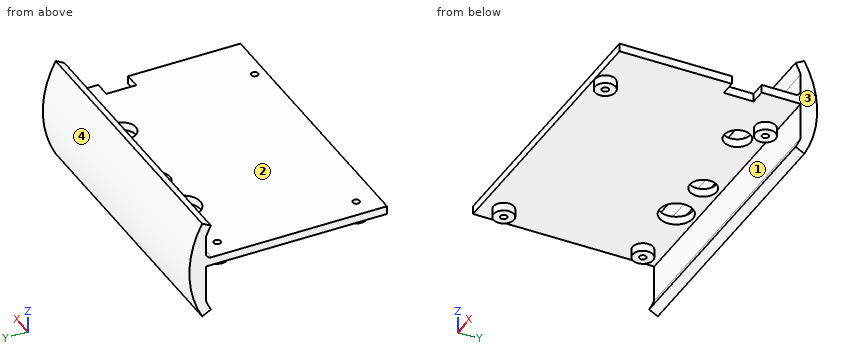
from build123d import *

# Parameters (mm, degrees)
ESBO_O1_R                                 = 5
ESBO_O1_R_2                               = 4
RESSALTO_EXTRUS_O4_DEPTH                  = 2.5
ESBO_O7_R                                 = 3.0875
RESSALTO_EXTRUS_O5_DEPTH                  = 2.5
BROCA_DE_ROSQUEAR_PARA_TARRAXA_DE_M2_51_D = 2.05
RESSALTO_EXTRUS_O6_REACH                  = 92.839


with BuildPart() as part:
    # Esboço1 → Ressalto-extrusão4 (new body)
    with BuildSketch(Plane.XY):
        Polygon((36.83, 26.550055291), (-30.48, 26.550055291), (-43.18, 26.550055291), (-43.18, 13.850055291), (-43.18, -15.359944709), (-43.18, -28.059944709), (-30.48, -28.059944709), (36.83, -28.059944709), (43.18, -28.059944709), (43.18, -21.709944709), (43.18, 5.794055291), (38.407682724, 5.794055291), (38.407682724, 14.794055291), (43.18, 14.794055291), (43.18, 20.200055291), (43.18, 26.550055291), align=None)
        with Locations((-18.322924579, 20.487241898)):
            Circle(ESBO_O1_R, mode=Mode.SUBTRACT)
        with Locations((-4.227566255, 21.406055391)):
            Circle(ESBO_O1_R_2, mode=Mode.SUBTRACT)
        with Locations((20.844433745, 18.879055391)):
            Circle(ESBO_O1_R_2, mode=Mode.SUBTRACT)
    extrude(amount=RESSALTO_EXTRUS_O4_DEPTH)

    # Esboço7 → Ressalto-extrusão5 (add)
    with BuildSketch(Plane(origin=(0, 0, 0), x_dir=(-1, 0, 0), z_dir=(0, 0, -1))):
        with Locations(Location((37.465, -21.709944709, 0), (0, 0, 180))):
            Circle(ESBO_O7_R)
        with Locations(Location((37.465, 20.200055291, 0), (0, 0, 180))):
            Circle(ESBO_O7_R)
        with Locations(Location((-28.575, 23.375055291, 0), (0, 0, 180))):
            Circle(ESBO_O7_R)
        with Locations(Location((-28.575, -24.884944709, 0), (0, 0, 180))):
            Circle(ESBO_O7_R)
    extrude(amount=RESSALTO_EXTRUS_O5_DEPTH)

    # Broca de rosquear para tarraxa de M2.51 (through all)
    with Locations(Plane(origin=(28.575, 23.375055291, -2.5), x_dir=(-1, 0, 0), z_dir=(0, 0, -1))):
        with Locations((0, 0), (66.04, -3.175), (0, -48.26), (66.04, -45.085)):
            Hole(BROCA_DE_ROSQUEAR_PARA_TARRAXA_DE_M2_51_D / 2)

    # Ressalto-extrusão6: up to this face of the body (flat: up to its plane)
    ressalto_extrus_o6_end = Plane(part.part.faces().sort_by_distance((43.18, 20.672055291, 1.25))[0])
    # Esboço9 → Ressalto-extrusão6 (add, up to the picked face)
    with BuildSketch(Plane.ZY.offset(43.18), mode=Mode.PRIVATE) as ressalto_extrus_o6_sk1:
        with BuildLine():
            Line((2.5, 24.836642303), (2.5, 26.550055291))
            Line((2.5, 26.550055291), (0, 26.550055291))
            Line((0, 26.550055291), (-11.160722179, 26.550055291))
            ThreePointArc((-11.160722179, 26.550055291), (-12.841855689, 25.831060984), (-14.473425786, 25.005747885))
            Line((-14.473425786, 25.005747885), (-15.912733763, 27.637931873))
            ThreePointArc((-15.912733763, 27.637931873), (-0.8, 31.5), (14.312733763, 27.637931873))
            Line((14.312733763, 27.637931873), (12.873425786, 25.005747885))
            ThreePointArc((12.873425786, 25.005747885), (11.241855689, 25.831060984), (9.560722179, 26.550055291))
            Line((9.560722179, 26.550055291), (4.213412987, 26.550055291))
            ThreePointArc((4.213412987, 26.550055291), (3.001847045, 26.048208246), (2.5, 24.836642303))
        make_face()
    ressalto_extrus_o6_tool1 = split(extrude(ressalto_extrus_o6_sk1.sketch, amount=-RESSALTO_EXTRUS_O6_REACH, mode=Mode.PRIVATE), bisect_by=ressalto_extrus_o6_end, keep=Keep.BOTH, mode=Mode.PRIVATE)
    add(ressalto_extrus_o6_tool1.solids().sort_by(Axis((-43.18, 28.43855, -0.780308), (1, 0, 0)))[0])


solid = part.part
Verification items for the finished model (mm, model axes). Face numbers are marked on the shaded views. Coordinates: 2 decimals unless noted, no trailing zeros. Write each loop counter-clockwise with the first axis right and the second up, starting at its lowest first coordinate (ties: lowest second). Pieces come first, ordered by that corner, then holes. Notation, with made-up numbers: (-36, 29) - (-23, 29) arc R24 ccw to (-23, 57) - close; hole circle Ø5 at (17.5, 73.25). An arc over 180 degrees is marked (long way). Answer as a JSON object with one key per item and string values.
(1) Cross-section at D-D on z = -6.5. Record the cut outline in (x, y).
Report:
{"outline": "(-43.18, 26.55) - (43.18, 26.55) - (43.18, 30.98) - (-43.18, 30.98) - close"}
(2) Thickness scan on line 1 along Y through (x, z) = (2.5, -1); line 2 along Z through (x, y) = (-5.5, 16.5); line 3 along Y through (x, z) = (37, -8). Record the ranges inside material, lowest first.
Report:
{"line 1": "26.55 to 31.5", "line 2": "0 to 2.5", "line 3": "26.55 to 30.67"}
(3) Cross-section at A-A on x = -19. Record the cut outline in (y, z), plus the area to 3 significant figures.
Report:
{"outline": "(-28.06, 0) - (15.53, 0) - (15.53, 2.5) - (-28.06, 2.5) - close; (24.84, 2.5) - (25.44, 2.5) - (25.44, 0) - (26.55, 0) - (26.55, -11.16) arc R28.5 cw to (25.01, -14.47) - (27.64, -15.91) arc R31.5 ccw to (27.64, 14.31) - (25.01, 12.87) arc R28.5 cw to (26.55, 9.56) - (26.55, 4.21) arc R1.71 cw to start", "area": "230 mm^2"}
(4) Cross-section at C-C on y = -1. Record the cut outline in (x, z), plus the area to 3 significant figures.
Report:
{"outline": "(-43.18, 0) - (43.18, 0) - (43.18, 2.5) - (-43.18, 2.5) - close", "area": "216 mm^2"}
(5) Mould release check, pull along Z, two halves, no side actions. Record for the marked faces 1, 2, 3 and 4: pulls with the +Z half, pulls with the -Z half, needs draft (parallel to the pull), parting line crosses it, or undercut.
Report:
{"face 1": "undercut", "face 2": "pulls with the +Z half", "face 3": "needs draft", "face 4": "parting line crosses it"}
(6) Gauge pin test, flat ends, axial feed: pin 1 Ø0.8 at (y, z) = (11, 1) entering from +X; pin 2 Ø4.5 at (x, z) = (-1, 7.5) entering from -Y; pin 3 Ø1.9 at (x, y) = (27.5, 24.5) entering from -Z. Record the tip position at first contact, or that the pin passes through.
Report:
{"pin 1": "x = 38.41", "pin 2": "y = 26.48", "pin 3": "z = -14.72"}
(7) Cross-section at B-B on x = 37. Record the cut outline in (y, z).
Report:
{"outline": "(-28.06, 0) - (26.55, 0) - (26.55, -11.16) arc R28.5 cw to (25.01, -14.47) - (27.64, -15.91) arc R31.5 ccw to (27.64, 14.31) - (25.01, 12.87) arc R28.5 cw to (26.55, 9.56) - (26.55, 4.21) arc R1.71 cw to (24.84, 2.5) - (-28.06, 2.5) - close"}
